from build123d import *

# Parameters (mm, degrees)
SKETCH1_R           = 1.6
BOSS_EXTRUDE1_DEPTH = 3


with BuildPart() as part:
    # Sketch1 → Boss-Extrude1 (new body)
    with BuildSketch(Plane.XY):
        Polygon((0, 145), (0, 0), (145, 0), (145, 15), (15, 145), align=None)
        with Locations((135, 7.5)):
            Circle(SKETCH1_R, mode=Mode.SUBTRACT)
        with Locations((110, 7.5)):
            Circle(SKETCH1_R, mode=Mode.SUBTRACT)
        with Locations((85, 7.5)):
            Circle(SKETCH1_R, mode=Mode.SUBTRACT)
        with Locations((60, 7.5)):
            Circle(SKETCH1_R, mode=Mode.SUBTRACT)
        with Locations((35, 7.5)):
            Circle(SKETCH1_R, mode=Mode.SUBTRACT)
        with Locations((7.5, 135)):
            Circle(SKETCH1_R, mode=Mode.SUBTRACT)
        with Locations((7.5, 110)):
            Circle(SKETCH1_R, mode=Mode.SUBTRACT)
        with Locations((7.5, 85)):
            Circle(SKETCH1_R, mode=Mode.SUBTRACT)
        with Locations((7.5, 60)):
            Circle(SKETCH1_R, mode=Mode.SUBTRACT)
        with Locations((7.5, 35)):
            Circle(SKETCH1_R, mode=Mode.SUBTRACT)
        Polygon((15, 123.418535773), (15, 15), (124.2033211, 15), align=None, mode=Mode.SUBTRACT)
    extrude(amount=BOSS_EXTRUDE1_DEPTH)


solid = part.part
Could you check a few things on this model? Use its own coordinates, in mm. A direction names the side the tool comes from. Coordinates: 2 decimals unless noted, no trailing zeros. Order: outer loops, then holes, each group sorted by start corner. A loop starts at its lowest first (then second) coordinate and runs counter-clockwise, first axis right, second up. Notation, with made-up numbers: (56, 86) -> (114, 86) arc R29 ccw to (114, 113) -> close; hole circle Ø2 at (-32.5, 73.5). An arc over 180 degrees is marked (long way). One line per question, with ' | ' between items.
Q1. Imagine slicing it at B-B on z = 1.35. State how many separate pieces and enclosed holes the cut face has, and give its area (3 significant figures).
Return value:
separate pieces: 1 | enclosed holes: 11 | area: 6,570 mm²
Q2. I'm going to push flat-ended pins straight in: P1, Ø1.5, axis at y = 82, z = 2, coming from the +X side; P2, Ø1.9, axis at x = 7.5, y = 110, coming from the -Z side; P3, Ø1, axis at y = 27, z = 1, coming from the +X side; P4, Ø1.5, axis at x = 87, z = 2, coming from the +Y side. Where does each tip first touch, or does it pass through?
Return value:
P1: x = 78.75 | P2: through | P3: x = 133.5 | P4: y = 73.75
Q3. Thinking about a two-plate mould opening in Y: for faces 1 (the face through (67, 73, 0)), 2 (the face through (81, 79, 1)), 3 (the face through (7.292, 61.586, 1.479)), which applies, pulls with the +Y half, pulls with the -Y half, needs draft (parallel to the pull), parting line crosses it, or undercut?
Return value:
face 1: needs draft | face 2: pulls with the +Y half | face 3: undercut
Q4. If I drill on L1, parallel to Y at x = 7.5, z = 2.35; L2, parallel to Y at x = 35, z = 2.4; L3, parallel to Y at x = 85, z = 2.05, over which ranges is the centre line in solid material (lowest first)?
Return value:
L1: 0 to 33.4, 36.6 to 58.4, 61.6 to 83.4, 86.6 to 108.4, 111.6 to 133.4, 136.6 to 145 | L2: 0 to 5.9, 9.1 to 15, 103.56 to 125 | L3: 0 to 5.9, 9.1 to 15, 53.92 to 75
Q5. Imagine slicing it at A-A on y = 76. Please give me the cut outline in (x, z).
Return value:
outline: (0, 0) -> (15, 0) -> (15, 3) -> (0, 3) -> close; (62.76, 0) -> (84, 0) -> (84, 3) -> (62.76, 3) -> close
Q6. Imagine slicing it at C-C on x = 31.5. Please give me the cut outline in (y, z).
Return value:
outline: (0, 0) -> (15, 0) -> (15, 3) -> (0, 3) -> close; (107.04, 0) -> (128.5, 0) -> (128.5, 3) -> (107.04, 3) -> close
Q7. On a 3-axis mill with a long thin cutter (end or side, diameter ignored), from which of +Z, -Z, +X, -X, +Y, -Y can I reach the whole of each face in a straight line? I mean faces 4 (the face through (67, 73, 3)), 5 (the face through (70.366, 68.45, 1.479)). Say none if no direction works.
Return value:
face 4: +Z, +X, -X, +Y, -Y | face 5: +Z, -Z
